```python
from build123d import *


with BuildPart() as f1:
    # F0 (on Front) → F1 (revolve)
    with BuildSketch(Plane.XZ):
        with BuildLine():
            Line((-43.328613, 0), (0, 0))
            Line((0, 0), (0, 1.5))
            Line((0, 1.5), (-41.958164, 1.5))
            ThreePointArc((-41.958164, 1.5), (-45.330697, 2.808655), (-46.937836, 6.04959))
            Line((-46.937836, 6.04959), (-63.029157, 183.952895))
            ThreePointArc((-63.029157, 183.952895), (-63.206857, 184.291819), (-63.572165, 184.405821))
            Line((-63.572165, 184.405821), (-64.070132, 184.36078))
            ThreePointArc((-64.070132, 184.36078), (-64.409056, 184.18308), (-64.523058, 183.817772))
            Line((-64.523058, 183.817772), (-48.308285, 4.54959))
            ThreePointArc((-48.308285, 4.54959), (-46.701145, 1.308655), (-43.328613, 0))
        make_face()
    revolve(axis=Axis((0, 0, 0.75), (0, 0, -1)))


solid = f1.part
```
The model under review builds one solid part; all positions refer to its coordinate system, in mm. A direction names the side the tool comes from. Round coordinates to 2 decimals unless told otherwise and drop trailing zeros. Loops run counter-clockwise (first coordinate to the right, second up) from the corner with the lowest first, then second, coordinate; pieces in that order, holes last.
Item 1: Take a section at A-A (y = 0). Write out the cut boundary in (x, z), then the cut area to 3 significant figures.
Determined:
outline: (-64.52, 183.82) - (-48.31, 4.55) arc R5 ccw to (-43.33, 0) - (43.33, 0) arc R5 ccw to (48.31, 4.55) - (64.52, 183.82) arc R0.5 ccw to (64.07, 184.36) - (63.57, 184.41) arc R0.5 ccw to (63.03, 183.95) - (46.94, 6.05) arc R5 cw to (41.96, 1.5) - (-41.96, 1.5) arc R5 cw to (-46.94, 6.05) - (-63.03, 183.95) arc R0.5 ccw to (-63.57, 184.41) - (-64.07, 184.36) arc R0.5 ccw to start
area: 695 mm2
Item 2: For faces 1 (the face through (-1, 1, 1.5)), 2 (the face through (1, 1, 0)), list the 3-axis set-ups (+Z, -Z, +X, -X, +Y, -Y) from which the entire face can be reached by the end or side of a thin tool; tool diameter is ignored.
Determined:
face 1: +Z
face 2: -Z, +X, -X, +Y, -Y
Item 3: Take a section at C-C (z = 69.5). Write out the cut boundary in (x, y), then the cut area to 3 significant figures.
Determined:
outline: circle Ø108.37 at (0, 0); hole circle Ø105.35 at (0, 0)
area: 506 mm2
Item 4: For line 1 (Z direction, x = 27, y = 18.5); line 2 (Y direction, x = 13, z = 38.5); line 3 (X direction, y = -5.5, z = 144), list the stretches that pass through material, from the lowest coordinate up.
Determined:
line 1: z = 0 to 1.5
line 2: y = -49.71 to -48.15, 48.15 to 49.71
line 3: x = -60.67 to -59.16, 59.16 to 60.67
Item 5: Clearance check with flat-ended pins moving along their axes: pin 1 Ø1.5 at (x, z) = (22, 132.5) entering from -Y; pin 2 Ø6 at (x, y) = (4.5, -40.5) entering from +Z; pin 3 Ø1.5 at (x, y) = (-6.5, -19.5) entering from +Z. State where each tip first meets the part, or that it passes through.
Determined:
pin 1: stops at y = -55.99
pin 2: stops at z = 1.83
pin 3: stops at z = 1.5
Item 6: Take a section at D-D (z = 122.5). Write out the cut boundary in (x, y).
Determined:
outline: circle Ø117.95 at (0, 0); hole circle Ø114.94 at (0, 0)
